The listing builds one solid part. Answer for the finished solid, in the listing's coordinates (mm). A direction names the side the tool comes from. Round coordinates to 2 decimals unless told otherwise and drop trailing zeros.
Item 1: This flat-tipped pin is pushed along its axis until it touches: pin 1 (2.5 mm diameter, centred on x = -135, z = -83, fed in from -Y). Where does it stop, or does it pass through?
Item 2: For a pull along Z with two mould halves and no side action, classify faces 1 (the face through (-135.268, 1.252, -154.644)), 2 (the face through (-94, 19, 0)), 3 (the face through (-94, 38.1, -119)) as +Z half, -Z half, draft (parallel to the pull), parting line (faces both ways), or undercut.
Item 3: A tool of negligible diameter and unlimited length cuts with its end or side. For faces 4 (the face through (-60, 2.54, -157)), 5 (the face through (-94, 0, -119)), from which of +Z, -Z, +X, -X, +Y, -Y can it reach the whole face along a straight path? Write none if from no direction.
Autodesk Inventor part; units mm, degrees
ref_plane "YZ Plane" through (0, 0, 0) normal (1, 0, 0) x (0, 1, 0)
ref_plane "XZ Plane" through (0, 0, 0) normal (0, 1, 0) x (-1, 0, 0)
ref_plane "XY Plane" through (0, 0, 0) normal (0, 0, 1) x (1, 0, 0)
sketch "Sketch1" plane through (0, 0, 0) normal (0, 1, 0) x (-1, 0, 0)
  line L0 (0, 0) -> (190.5, 0)
  line L1 (190.5, 0) -> (190.5, -241.3)
  line L2 (190.5, -241.3) -> (0, -241.3)
  line L3 (0, -241.3) -> (0, 0)
  dimension "d0" = 190.5
  dimension "d1" = 241.3
extrude "Extrusion1" add sketch "Sketch1" along normal blind 38.1
sketch "Sketch2" plane through (0, 0, 0) normal (0, -1, 0) x (1, 0, 0)
  circle A0 centre (-134.9375, -157.1625) radius 2.54
  line L0 (-190.5, 0) -> (-190.5, -241.3)
  line L1 (0, -241.3) -> (-190.5, -241.3)
  circle A1 centre (-60.325, -157.1625) radius 2.54
  circle A2 centre (-134.9375, -82.55) radius 2.54
  circle A3 centre (-60.325, -82.55) radius 2.54
  point P0 (0, 0)
  dimension "d4" = 5.08
  dimension "d5" = 55.5625
  dimension "d6" = 84.1375
  dimension "d7" = 5.08
  dimension "d8" = 5.08
  dimension "d9" = 74.6125
  dimension "d10" = 74.6125
  dimension "d11" = 5.08
  dimension "d12" = 74.6125
  dimension "d13" = 74.6125
extrude "Extrusion2" cut sketch "Sketch2" against normal blind 2.54
properties part number "screen"
Check values:
1. pin 1: stops at y = 2.54
2. face 1: undercut
2. face 2: +Z half
2. face 3: draft
3. face 4: -Y
3. face 5: +Z, -Z, +X, -X, -Y
